```python
from build123d import *

# Parameters (mm, degrees)
SKETCH_1_W               = 119
SKETCH_1_H               = 62
EXTRUDE_1_DEPTH          = 8
CUT_EXTRUDE_1_REACH      = 360.247
HOLE_WIZARD_M5_1_D       = 5.3
SKETCH_11_W              = 119
SKETCH_11_H              = 11.469825071
CUT_EXTRUDE_5_DEPTH      = 359.24680204
PATTERN_CIRCULAR_1_COUNT = 3
CUT_EXTRUDE_2_DEPTH      = 359.24680204
CUT_EXTRUDE_2_DEPTH_BACK = 359.24680204
SKETCH_7_W               = 46
SKETCH_7_H               = 140
CUT_EXTRUDE_4_DEPTH      = 359.24680204
HOLE_WIZARD_M6_1_D       = 6.4
CUT_EXTRUDE_6936_REACH   = 360.247
SKETCH_10_R              = 60
FILLET_4_R               = 8
HOLE_WIZARD_M4_1_D       = 3.3
HOLE_WIZARD_M3_1_D       = 3.2
HOLE_WIZARD_9_0_9_1_D    = 9
CUT_EXTRUDE_6_DEPTH      = 10
HOLE_WIZARD_M3_3_D       = 3.4


with BuildPart() as part:
    # 草图1 → 凸台-拉伸1 (new body)
    with BuildSketch(Plane(origin=(0, 0, 0), x_dir=(1, 0, 0), z_dir=(0, 1, 0))):
        Polygon((-182.426223927, 186.923957016), (-250, 69.882743599), (-241.006855494, 20.698159104), (-105.890151719, -222.811211717), (-68.915866776, -256.469825071), (68.915866776, -256.469825071), (105.890151719, -222.811211717), (241.006855494, 20.698159104), (250, 69.882743599), (182.426223927, 186.923957016), (129.416945427, 230), (-129.416945427, 230), align=None)
        Polygon((188.232648893, 39.971488475), (128.732648893, 143.028511525), (182.426223927, 174.028511525), (241.926223927, 70.971488475), align=None, mode=Mode.SUBTRACT)
        Polygon((-128.732648893, 143.028511525), (-188.232648893, 39.971488475), (-241.926223927, 70.971488475), (-182.426223927, 174.028511525), align=None, mode=Mode.SUBTRACT)
        with Locations((0, -214)):
            Rectangle(SKETCH_1_W, SKETCH_1_H, mode=Mode.SUBTRACT)
    extrude(amount=EXTRUDE_1_DEPTH)

    # 草图2 → 切除-拉伸1 (cut, up to next)
    with BuildSketch(Plane(origin=(0, 8, 0), x_dir=(1, 0, 0), z_dir=(0, 1, 0)), mode=Mode.PRIVATE) as cut_extrude_1_sk1:
        Polygon((-124.851251684, 39.751288694), (-96.851251684, 88.248711306), (-144.482648893, 115.748711306), (-172.482648893, 67.251288694), align=None)
    cut_extrude_1_tool1 = extrude(cut_extrude_1_sk1.sketch, amount=-CUT_EXTRUDE_1_REACH, mode=Mode.PRIVATE) & part.part
    cut_extrude_1 = cut_extrude_1_tool1.solids().sort_by_distance((-134.66695, 8, -77.75))[0]
    add(cut_extrude_1, mode=Mode.SUBTRACT)

    # M5 间隙孔1 (through all)
    with Locations(Plane(origin=(0, 8, 0), x_dir=(-1, 0, 0), z_dir=(0, 1, 0))):
        with Locations((106.225607337, -100.011851027), (137.402521874, -118.011851027), (139.725607337, -41.988148973), (170.902521874, -59.988148973)):
            hole_wizard_m5_1 = Hole(HOLE_WIZARD_M5_1_D / 2)

    # 草图11 → 切除-拉伸5 (cut, through all)
    with BuildSketch(Plane(origin=(0, 8, 0), x_dir=(1, 0, 0), z_dir=(0, 1, 0))):
        Polygon((182.426223927, 174.028511525), (241.926223927, 70.971488475), (247.510115621, 74.195349848), (188.010115621, 177.252372898), align=None)
        with Locations((0, -250.734912536)):
            Rectangle(SKETCH_11_W, SKETCH_11_H)
        Polygon((-241.926223927, 70.971488475), (-182.426223927, 174.028511525), (-188.010115621, 177.252372898), (-247.510115621, 74.195349848), align=None)
    extrude(amount=-CUT_EXTRUDE_5_DEPTH, mode=Mode.SUBTRACT)

    # 阵列(圆周)1: 切除-拉伸1, M5 间隙孔1 ×3 about axis
    pattern_circular_1_axis = Axis((0, 0, 0), (0, 1, 0))
    add([cut_extrude_1.rotate(pattern_circular_1_axis, i * 360 / PATTERN_CIRCULAR_1_COUNT) for i in range(1, PATTERN_CIRCULAR_1_COUNT)], mode=Mode.SUBTRACT)
    add([hole_wizard_m5_1.rotate(pattern_circular_1_axis, i * 360 / PATTERN_CIRCULAR_1_COUNT) for i in range(1, PATTERN_CIRCULAR_1_COUNT)], mode=Mode.SUBTRACT)

    # 草图5 → 切除-拉伸2 (cut, two sides: drawn at the far end of the back side and taken through both)
    with BuildSketch(Plane(origin=(0, 8, 0), x_dir=(1, 0, 0), z_dir=(0, 1, 0)).offset(-CUT_EXTRUDE_2_DEPTH_BACK)):
        Polygon((35, 145), (120, 230), (-120, 230), (-35, 145), align=None)
    extrude(amount=CUT_EXTRUDE_2_DEPTH + CUT_EXTRUDE_2_DEPTH_BACK, mode=Mode.SUBTRACT)

    # 草图7 → 切除-拉伸4 (cut, through all)
    with BuildSketch(Plane(origin=(0, 8, 0), x_dir=(1, 0, 0), z_dir=(0, 1, 0))):
        with Locations((0, 160)):
            Rectangle(SKETCH_7_W, SKETCH_7_H)
    extrude(amount=-CUT_EXTRUDE_4_DEPTH, mode=Mode.SUBTRACT)

    # M6 间隙孔1 (through all)
    with Locations(Plane(origin=(0, 8, 0), x_dir=(1, 0, 0), z_dir=(0, 1, 0))):
        with Locations((30, 114.64), (-30, 114.64)):
            Hole(HOLE_WIZARD_M6_1_D / 2)

    # 草图10 → Cut-Extrude 6936 (cut, up to next)
    with BuildSketch(Plane(origin=(0, 8, 0), x_dir=(1, 0, 0), z_dir=(0, 1, 0)), mode=Mode.PRIVATE) as cut_extrude_6936_sk1:
        with Locations(Location((0, 0, 0), (0, 0, 270))):
            Circle(SKETCH_10_R)
    cut_extrude_6936_tool1 = extrude(cut_extrude_6936_sk1.sketch, amount=-CUT_EXTRUDE_6936_REACH, mode=Mode.PRIVATE) & part.part
    add(cut_extrude_6936_tool1.solids().sort_by_distance((0, 8, 0))[0], mode=Mode.SUBTRACT)

    # 圆角4
    fillet_4_edges = [part.edges().sort_by_distance(p)[0] for p in [
        (-128.732648893, 4, -143.028511525),
        (-188.232648893, 4, -39.971488475),
        (188.232648893, 4, -39.971488475),
        (128.732648893, 4, -143.028511525),
        (-59.5, 4, 183),
        (59.5, 4, 183),
    ]]
    fillet(fillet_4_edges, radius=FILLET_4_R)

    # M4 螺纹孔1 (through all)
    with Locations(Plane(origin=(0, 8, 0), x_dir=(1, 0, 0), z_dir=(0, 1, 0))):
        with Locations((-79, -0.36), (79, -0.36)):
            Hole(HOLE_WIZARD_M4_1_D / 2)

    # M3 间隙孔1 (through all)
    with Locations(Plane(origin=(0, 0, 0), x_dir=(-1, 0, 0), z_dir=(0, -1, 0))):
        with Locations((-121.660848414, -75.343344122), (-70.91, -145.125228485), (-137.200449982, -123.918242815), (-55.370398432, -96.550329791)):
            hole_wizard_m3_1 = Hole(HOLE_WIZARD_M3_1_D / 2)

    # Ø9.0 (9) 直径孔1 (through all)
    with Locations(Plane(origin=(0, 0, 0), x_dir=(-1, 0, 0), z_dir=(0, -1, 0))):
        with Locations((-105.902393669, -94.348635597), (-79.233821838, -102.880181556)):
            hole_wizard_9_0_9_1 = Hole(HOLE_WIZARD_9_0_9_1_D / 2)

    # 草图21 → 切除-拉伸6 (cut)
    with BuildSketch(Plane.XZ):
        Polygon((88.85332577, 149.359264422), (92.509702609, 160.78865235), (128.702764381, 149.210125692), (125.046387542, 137.780737764), align=None)
    cut_extrude_6 = extrude(amount=-CUT_EXTRUDE_6_DEPTH, mode=Mode.SUBTRACT)

    # M3 间隙孔3 (through all)
    with Locations(Plane(origin=(0, 0, 0), x_dir=(-1, 0, 0), z_dir=(0, -1, 0))):
        with Locations((53.517161568, 137.386324493), (78.508936531, 147.604503599)):
            hole_wizard_m3_3 = Hole(HOLE_WIZARD_M3_3_D / 2)

    # 镜向1: M3 间隙孔1, Ø9.0 (9) 直径孔1, 切除-拉伸6, M3 间隙孔3 across plane
    add(hole_wizard_m3_1.mirror(Plane(origin=(0, 0, 0), x_dir=(0, 0, 1), z_dir=(1, 0, 0))), mode=Mode.SUBTRACT)
    add(hole_wizard_9_0_9_1.mirror(Plane(origin=(0, 0, 0), x_dir=(0, 0, 1), z_dir=(1, 0, 0))), mode=Mode.SUBTRACT)
    add(cut_extrude_6.mirror(Plane(origin=(0, 0, 0), x_dir=(0, 0, 1), z_dir=(1, 0, 0))), mode=Mode.SUBTRACT)
    add(hole_wizard_m3_3.mirror(Plane(origin=(0, 0, 0), x_dir=(0, 0, 1), z_dir=(1, 0, 0))), mode=Mode.SUBTRACT)


solid = part.part
```
Input: part model. Units: mm. Frame: model coordinates. A direction names the side the tool comes from. Give positions to 0.01 mm unless a question says otherwise; leave off trailing zeros. Loops run counter-clockwise (first coordinate to the right, second up) from the corner with the lowest first, then second, coordinate; pieces in that order, holes last.
1) Section query A-A on y = 3. Count the separate pieces of the cut face and the enclosed holes in it, and give its area (3 significant figures).
A:
separate pieces: 1
enclosed holes: 35
area: 116,000 mm2
2) Contact query for flat-ended pins moving along their axis: pin 1 (4 mm diameter, centred on x = 29, y = 3.5, fed in from -Z); pin 2 (7 mm diameter, centred on x = 170.9, z = -59.99, fed in from +Y); pin 3 (2.5 mm diameter, centred on y = 3, z = 208, fed in from +X); pin 4 (1 mm diameter, centred on y = 2.5, z = -134.5, fed in from +X). Output: stop coordinate, or through.
A:
pin 1: stops at z = -145
pin 2: stops at y = 8
pin 3: stops at x = 114.8
pin 4: stops at x = 133.95
3) Mould query, pull axis X, two halves, no side actions, for faces 6 (the flat face through (-87.662, 3.944, 239.405)), 7 (the flat face through (77, 4, -187)), 8 (the flat face through (156.293, 3.944, -208.16)). Classes: released by +X, released by -X, zero draft, split by the parting line, or undercut.
A:
face 6: released by -X
face 7: undercut
face 8: released by +X
4) Line query: L1, parallel to Z at x = -30, y = 4.75; L2, parallel to Z at x = 33.5, y = 4.5; L3, parallel to X at y = 5, z = 122.5. Output: solid intervals per line, ascending.
A:
L1: z = -145 to -117.84, -111.44 to -51.96, 51.96 to 183
L2: z = -145 to -49.78, 49.78 to 139.35, 144.65 to 175.35, 180.65 to 183
L3: x = -161.55 to -137.94, -136.46 to 136.46, 137.94 to 161.55
5) Section query B-B on x = 213. Return the cut outline in (y, z), and give its area (3 significant figures).
A:
outline: (0, -54.27) - (8, -54.27) - (8, 29.78) - (0, 29.78) - close
area: 672 mm2
6) Reachability of faces 1 (the flat face through (-138.525, 3.944, -126.067)), 2 (the flat face through (178.44, 3.94, -56.93)), 3 (the flat face through (138.69, 3.94, -125.78)), 4 (the flat face through (-78, 4, -188)), 5 (the flat face through (-174.394, 3.944, 99.352)) from +Z, -Z, +X, -X, +Y, -Y: full face, straight path, thin tool, end or side. Return the list, or none.
A:
face 1: -X, +Y, -Y
face 2: +Y, -Y
face 3: +X, +Y, -Y
face 4: -Z, +Y, -Y
face 5: +Z, -X, +Y, -Y
